Geometry check sheet. Reference: the model listing, model coordinates, mm. Face numbers are marked on the shaded views. Give positions to 0.01 mm unless a question says otherwise; leave off trailing zeros. Order: outer loops, then holes, each group sorted by start corner. A loop starts at its lowest first (then second) coordinate and runs counter-clockwise, first axis right, second up.
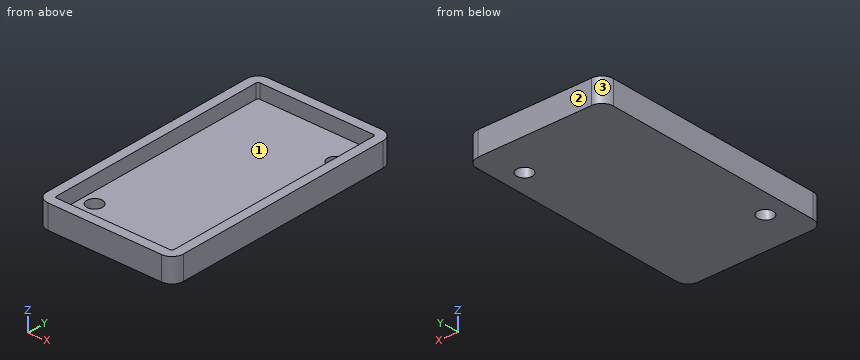
from build123d import *

# Parameters (mm, degrees)
F0_W     = 28.75
F0_H     = 51.8
F1_DEPTH = 5
F2_R     = 2.4142135624
F3_T     = -2
F4_D     = 3.3


with BuildPart() as f1:
    # F0 (on Top) → F1 (new body)
    with BuildSketch(Plane.XY):
        Rectangle(F0_W, F0_H)
    extrude(amount=F1_DEPTH)

    # F2
    f2_edges = [f1.edges().sort_by_distance(p)[0] for p in [
        (14.375, -25.9, 2.5),
        (-14.375, -25.9, 2.5),
        (14.375, 25.9, 2.5),
        (-14.375, 25.9, 2.5),
    ]]
    fillet(f2_edges, radius=F2_R)

    # F3
    f3_openings = [f1.faces().sort_by_distance(p)[0] for p in [
        (0, 0, 5),
    ]]
    offset(amount=F3_T, openings=f3_openings)

    # F4 (through all)
    with Locations(Plane(origin=(0, 0, 0), x_dir=(1, 0, 0), z_dir=(0, 0, -1))):
        with Locations((9.725, -17.46), (-9.725, 17.46)):
            Hole(F4_D / 2)


solid = f1.part
Item 1: Sectioned sample at A-A (y = -17.46). Enter the section's corners in (x, z) (3 decimals).
Reported:
outline: (-14.375, 0) - (-11.375, 0) - (-11.375, 2) - (-12.375, 2) - (-12.375, 5) - (-14.375, 5) - close; (-8.075, 0) - (14.375, 0) - (14.375, 5) - (12.375, 5) - (12.375, 2) - (-8.075, 2) - close
Item 2: Sectioned sample at B-B (z = 4.45). Enter the section's corners in (x, y) (3 decimals).
Reported:
outline: (-14.375, -23.486) arc R2.414 ccw to (-11.961, -25.9) - (11.961, -25.9) arc R2.414 ccw to (14.375, -23.486) - (14.375, 23.486) arc R2.414 ccw to (11.961, 25.9) - (-11.961, 25.9) arc R2.414 ccw to (-14.375, 23.486) - close; hole (-12.375, -23.486) arc R0.414 ccw to (-11.961, -23.9) - (11.961, -23.9) arc R0.414 ccw to (12.375, -23.486) - (12.375, 23.486) arc R0.414 ccw to (11.961, 23.9) - (-11.961, 23.9) arc R0.414 ccw to (-12.375, 23.486) - close
Item 3: Draft check along X on the marked faces 1, 2 and 3. Enter one of: released by +X, released by -X, zero draft, split by the parting line, or undercut.
Reported:
face 1: undercut
face 2: zero draft
face 3: released by -X
Item 4: Scan lines: L1, parallel to X at y = 14.5, z = 3.7 (3 decimals); L2, parallel to Y at x = 6.5, z = 2.5; L3, parallel to X at y = -17.46, z = 1.1 (3 decimals). Record each from-to range of solid material in increasing order.
Reported:
L1: x = -14.375 to -12.375, 12.375 to 14.375
L2: y = -25.9 to -23.9, 23.9 to 25.9
L3: x = -14.375 to -11.375, -8.075 to 14.375
Item 5: Sectioned sample at D-D (y = 18). Enter the section's corners in (x, z) (3 decimals).
Reported:
outline: (-14.375, 0) - (8.166, 0) - (8.166, 2) - (-12.375, 2) - (-12.375, 5) - (-14.375, 5) - close; (11.284, 0) - (14.375, 0) - (14.375, 5) - (12.375, 5) - (12.375, 2) - (11.284, 2) - close
Item 6: Sectioned sample at C-C (x = 0.5). Enter the section's corners in (y, z).
Reported:
outline: (-25.9, 0) - (25.9, 0) - (25.9, 5) - (23.9, 5) - (23.9, 2) - (-23.9, 2) - (-23.9, 5) - (-25.9, 5) - close
Item 7: Gauge pin test, flat ends, axial feed: pin 1 (2 mm diameter, centred on x = -3, y = 8.5, fed in from +Z); pin 2 (1.5 mm diameter, centred on x = 2.5, y = 19, fed in from -Z). Record the tip position at first contact, or that the pin passes through.
Reported:
pin 1: stops at z = 2
pin 2: stops at z = 0
